The listing builds one solid part. Answer for the finished solid, in the listing's coordinates (mm). Face numbers are marked on the shaded views. A direction names the side the tool comes from. Give positions to 0.01 mm unless a question says otherwise; leave off trailing zeros. Loops run counter-clockwise (first coordinate to the right, second up) from the corner with the lowest first, then second, coordinate; pieces in that order, holes last. Notation, with made-up numbers: (-33.5, 43.25) - (-21.5, 43.25) arc R12 cw to (-21.5, 51.25) - close; hole circle Ø5 at (47, -13.5). An arc over 180 degrees is marked (long way). Write item = value, one per line. Start each with the question number.
1) The mould has two halves that part along Z. Classify the marked faces 1, 2 and 3: +Z half, -Z half, draft (parallel to the pull), parting line (faces both ways), or undercut.
2) Consider probe 1 along X at (y, z) = (4.3, 0); probe 2 along Z at (x, y) = (0, 4.35); probe 3 along Y at (x, z) = (1.25, 2.75). Determine where each line is inside the solid, lowest interval first.
3) The part is cut by section C-C on z = 2.25. Write down the section's boundary in (x, y), plus the area to 3 significant figures.
4) The part is cut by section D-D on y = 7. Write down the section's boundary in (x, z).
5) Flat-ended cylindrical pins translate along their axes: P1, Ø1.8, axis at x = -1.5, y = 6, coming from the +Z side; P2, Ø1.8, axis at y = 2, z = -2, coming from the -X side; P3, Ø3, axis at x = 0, z = -2.5, coming from the -Y side. Find the tip coordinate at first contact, or state that the pin passes through.
6) The part is cut by section B-B on y = 1. Write down the section's boundary in (x, z).
7) The part is cut by section A-A on x = 0. Write down the section's boundary in (y, z).
8) Which of the six approach directions +Z, -Z, +X, -X, +Y, -Y give full straight-line access (tool end or side, diameter ignored) to the marked faces 4, 5 and 6?
from build123d import *

# Parameters (mm, degrees)
SKETCH1_R           = 1.5
BOSS_EXTRUDE1_DEPTH = 8
SKETCH2_W           = 2
SKETCH2_H           = 2
SKETCH2_H_2         = 4
SKETCH2_W_2         = 6
CUT_EXTRUDE1_DEPTH  = 9
SKETCH3_W           = 3
SKETCH3_H           = 3
CUT_EXTRUDE2_DEPTH  = 18


with BuildPart() as part:
    # Sketch1 → Boss-Extrude1 (new body)
    with BuildSketch(Plane(origin=(0, 0, 0), x_dir=(1, 0, 0), z_dir=(0, 1, 0))):
        with BuildLine():
            Line((-3, -4), (-3, -3))
            Line((-3, -3), (3, -3))
            Line((3, -3), (3, -4))
            ThreePointArc((3, -4), (0, 5), (-3, -4))
        make_face()
        Circle(SKETCH1_R, mode=Mode.SUBTRACT)
    extrude(amount=BOSS_EXTRUDE1_DEPTH)

    # Sketch2 → Cut-Extrude1 (cut, symmetric)
    with BuildSketch(Plane.XY):
        with Locations((4, 7)):
            Rectangle(SKETCH2_W, SKETCH2_H)
        with Locations((-4, 6)):
            Rectangle(SKETCH2_W, SKETCH2_H_2)
        with Locations((0, 1)):
            Rectangle(SKETCH2_W_2, SKETCH2_H)
    extrude(amount=CUT_EXTRUDE1_DEPTH, both=True, mode=Mode.SUBTRACT)

    # Sketch3 → Cut-Extrude2 (cut)
    with BuildSketch(Plane.XY):
        with Locations((0, 6.5)):
            Rectangle(SKETCH3_W, SKETCH3_H)
    extrude(amount=CUT_EXTRUDE2_DEPTH, mode=Mode.SUBTRACT)


solid = part.part
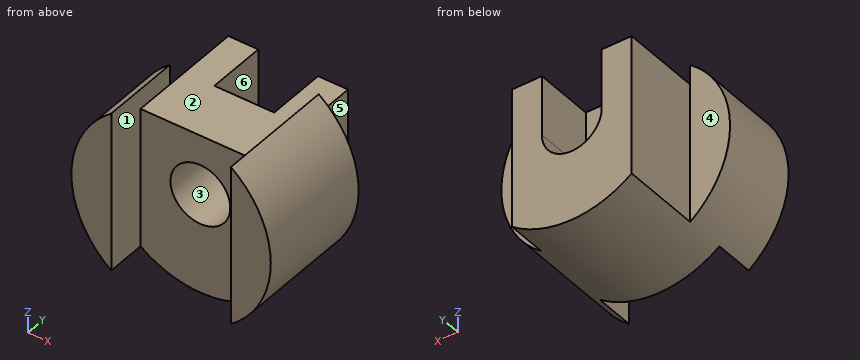
Answer below:
q1.face_1 = draft
q1.face_2 = +Z half
q1.face_3 = undercut
q2.probe_1 = -3 to -1.5, 1.5 to 5
q2.probe_2 = -5 to -1.5, 1.5 to 3
q2.probe_3 = 2 to 5
q3.outline = (-4.47, 0) - (-3, 0) - (-3, 2) - (3, 2) - (3, 0) - (4.47, 0) - (4.47, 6) - (3, 6) - (3, 8) - (1.5, 8) - (1.5, 5) - (-1.5, 5) - (-1.5, 8) - (-3, 8) - (-3, 4) - (-4.47, 4) - close
q3.area = 41.7 mm2
q4.outline = (-3, -4) arc R5 ccw to (3, -4) - (3, 3) - (1.5, 3) - (1.5, 0) arc R1.5 cw to (-1.5, 0) - (-1.5, 3) - (-3, 3) - close
q5.P1 = 3
q5.P2 = -4.88
q5.P3 = 2
q6.outline = (-3, -4) - (-3, 4) arc R5 ccw to start; (3, -4) arc R5 ccw to (3, 4) - close
q7.outline = (2, -5) - (8, -5) - (8, -1.5) - (2, -1.5) - close; (2, 1.5) - (5, 1.5) - (5, 3) - (2, 3) - close
q8.face_4 = +Z, -Z, -X, +Y
q8.face_5 = +Z, -Z, +X, +Y
q8.face_6 = +Z, +Y
